Read the model definition and answer for the solid it produces. Units are mm, in the model's axes. Round coordinates to 2 decimals unless told otherwise and drop trailing zeros. Write each loop counter-clockwise with the first axis right and the second up, starting at its lowest first coordinate (ties: lowest second). Pieces come first, ordered by that corner, then holes. Notation, with made-up numbers: (4, 38.5) -> (33, 38.5) arc R27 cw to (33, 56.5) -> close; hole circle Ø8 at (-23.75, -15). An arc over 180 degrees is marked (long way). Return JSON: item names as keys, results as strings.
from build123d import *

# Parameters (mm, degrees)
F1_DEPTH = 25


with BuildPart() as f1:
    # F0 (on Front) → F1 (new body)
    with BuildSketch(Plane.XZ):
        with BuildLine():
            Line((-41.461691, -10.433468), (41.461691, -10.433468))
            Line((41.461691, -10.433468), (41.461691, 10.433468))
            Line((41.461691, 10.433468), (35.64515, 10.433468))
            ThreePointArc((35.64515, 10.433468), (37.250754, 8.513963), (37.826613, 6.078629))
            ThreePointArc((37.826613, 6.078629), (29.953782, 1.216991), (29.133081, 10.433468))
            Line((29.133081, 10.433468), (17.131031, 10.433468))
            ThreePointArc((17.131031, 10.433468), (18.736635, 8.513963), (19.312494, 6.078629))
            ThreePointArc((19.312494, 6.078629), (11.439663, 1.216991), (10.618963, 10.433468))
            Line((10.618963, 10.433468), (-10.618963, 10.433468))
            ThreePointArc((-10.618963, 10.433468), (-9.013358, 8.513963), (-8.437499, 6.078629))
            ThreePointArc((-8.437499, 6.078629), (-16.310331, 1.216991), (-17.131031, 10.433468))
            Line((-17.131031, 10.433468), (-29.133081, 10.433468))
            ThreePointArc((-29.133081, 10.433468), (-27.527477, 8.513963), (-26.951618, 6.078629))
            ThreePointArc((-26.951618, 6.078629), (-34.824449, 1.216991), (-35.64515, 10.433468))
            Line((-35.64515, 10.433468), (-41.461691, 10.433468))
            Line((-41.461691, 10.433468), (-41.461691, -10.433468))
        make_face()
    extrude(amount=F1_DEPTH)


solid = f1.part
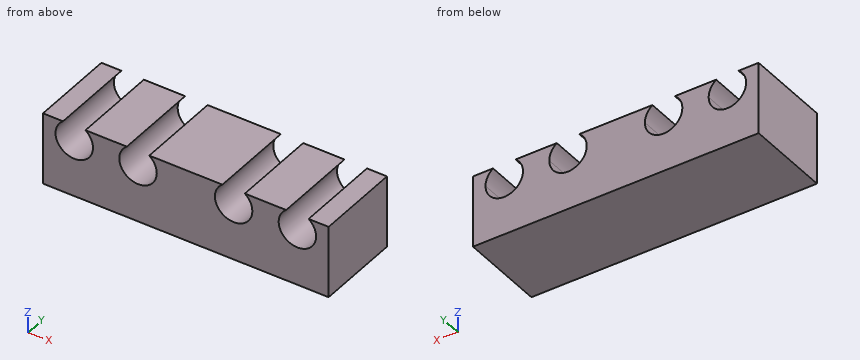
Item 1: Section A-A (z = 3) is taken. Give the vertices of the cut face in (x, y), then the cut area to 3 significant figures.
Worked answers:
{"outline": "(-41.46, -25) -> (-36.87, -25) -> (-36.87, 0) -> (-41.46, 0) -> close; (-27.91, -25) -> (-18.36, -25) -> (-18.36, 0) -> (-27.91, 0) -> close; (-9.39, -25) -> (9.39, -25) -> (9.39, 0) -> (-9.39, 0) -> close; (18.36, -25) -> (27.91, -25) -> (27.91, 0) -> (18.36, 0) -> close; (36.87, -25) -> (41.46, -25) -> (41.46, 0) -> (36.87, 0) -> close", "area": "1,180 mm2"}
Item 2: Section C-C (x = 18) is taken. Give the vertices of the cut face in (y, z), then the cut area to 3 significant figures.
Worked answers:
{"outline": "(-25, -10.43) -> (0, -10.43) -> (0, 2.54) -> (-25, 2.54) -> close; (-25, 9.62) -> (0, 9.62) -> (0, 10.43) -> (-25, 10.43) -> close", "area": "345 mm2"}
Item 3: A flat-ended cylindrical pin translates along its axis: pin 1 (10 mm diameter, centred on x = 32.39, z = 6.08, fed in from -Y). Find the tip coordinate at first contact, or state that the pin passes through.
Worked answers:
{"pin 1": "passes through"}
Item 4: Straight lines are drawn through the part: L1, parallel to X at y = -10.75, z = 5.75; L2, parallel to X at y = -6, z = 6.5; L3, parallel to Z at x = 37, y = -17.75. For each, find the intervals that lie inside material, in ascending order. Write a range as [from, to].
Worked answers:
{"L1": "x = [-41.46, -37.82], [-26.96, -19.3], [-8.45, 8.45], [19.3, 26.96], [37.82, 41.46]", "L2": "x = [-41.46, -37.81], [-26.97, -19.3], [-8.45, 8.45], [19.3, 26.97], [37.81, 41.46]", "L3": "z = [-10.43, 3.2], [8.96, 10.43]"}
Item 5: Section D-D (x = -15.5) is taken. Give the vertices of the cut face in (y, z).
Worked answers:
{"outline": "(-25, -10.43) -> (0, -10.43) -> (0, 0.89) -> (-25, 0.89) -> close"}
Item 6: Section B-B (y = -7) is taken. Give the vertices of the cut face in (x, z) (1 decimal), then the cut area to 3 significant figures.
Worked answers:
{"outline": "(-41.5, -10.4) -> (41.5, -10.4) -> (41.5, 10.4) -> (35.6, 10.4) arc R5.4 cw (long way) to (29.1, 10.4) -> (17.1, 10.4) arc R5.4 cw (long way) to (10.6, 10.4) -> (-10.6, 10.4) arc R5.4 cw to (-8.4, 6.1) arc R5.4 cw (long way) to (-17.1, 10.4) -> (-29.1, 10.4) arc R5.4 cw (long way) to (-35.6, 10.4) -> (-41.5, 10.4) -> close", "area": "1,380 mm2"}
